The listing builds one solid part. Answer for the finished solid, in the listing's coordinates (mm). A direction names the side the tool comes from. Coordinates: 2 decimals unless noted, no trailing zeros. Loops run counter-clockwise (first coordinate to the right, second up) from the corner with the lowest first, then second, coordinate; pieces in that order, holes last. Notation, with made-up numbers: M 64.25,-20.5 L 94.25,-20.5 A6 ccw 94.25,-13.5 Z; hole C 83,63.5 d10. An arc over 180 degrees is marked long. Return JSON: item names as keys, results as strings. Group by question number.
1. Section B-B (z = -2.25) is taken. Count the separate pieces of the cut face and the enclosed holes in it, then the cut area to 3 significant figures.
2. Section A-A (y = 5.5) is taken. Write down the section's boundary in (x, z), then the cut area to 3 significant figures.
3. Given P1, Ø6, axis at x = -1, y = 7, coming from the -Z side; P2, Ø2.5, axis at y = 0, z = -3, coming from the +X side; P3, Ø0.5, axis at x = 7, z = -2, coming from the +Y side, each flat-ended and moving along its own axis, determine where each tip first touches the part or whether it passes through.
4. Straight lines are drawn through the part: L1, parallel to X at y = 2, z = -0.25; L2, parallel to Y at x = 6.25, z = 0.5; L3, parallel to X at y = 0.5, z = -0.5. For each, find the intervals that lie inside material, in ascending order. Write a range as from..to.
5. Section D-D (z = 1.25) is taken. Write down the section's boundary in (x, y), then the cut area to 3 significant figures.
6. Which of the six approach directions +Z, -Z, +X, -X, +Y, -Y give full straight-line access (tool end or side, diameter ignored) to faces 1 (the face through (-4, 0, -1)), 2 (the face through (0, 0, 2.5))?
7. The mould has two halves that part along X. Classify faces 3 (the face through (1.143, 1.121, -6.207)), 4 (the face through (9, -0.1, 0.4)), 5 (the face through (-1.121, 1.143, -6.207)): pulls with the +X half, pulls with the -X half, needs draft (parallel to the pull), parting line crosses it, or undercut.
```python
from build123d import *

# Parameters (mm, degrees)
SKETCH1_W               = 20
SKETCH1_H               = 20
BOSS_EXTRUDE1_DEPTH     = 2.5
BOSS_EXTRUDE1_TAPER     = 15
SKETCH2_W               = 18
SKETCH2_H               = 18
CUT_EXTRUDE1_DEPTH      = 0.85
SKETCH3_R               = 2
BOSS_EXTRUDE2_DEPTH     = 8.2
BOSS_EXTRUDE2_TAPER     = 1.5
CHAMFER1_SIZE           = 2
CHAMFER1_SIZE_2         = 0.5
FILLET1_R               = 0.5
SKETCH4_W               = 0.5
SKETCH4_H               = 6.160058372
SKETCH4_W_2             = 6.292216955
SKETCH4_H_2             = 0.5
CUT_EXTRUDE_THIN1_DEPTH = 8.2
CUT_EXTRUDE_THIN1_TAPER = 1
BOSS_EXTRUDE3_DEPTH     = 5
FILLET2_R               = 1
FILLET3_R               = 0.75
CUT_EXTRUDE2_DEPTH      = 5
FILLET2_OF_MIRROR1_R    = 1
FILLET3_OF_MIRROR1_R    = 0.75


with BuildPart() as part:
    # Sketch1 → Boss-Extrude1 (new body)
    with BuildSketch(Plane.XY):
        Rectangle(SKETCH1_W, SKETCH1_H)
    extrude(amount=BOSS_EXTRUDE1_DEPTH, taper=BOSS_EXTRUDE1_TAPER)

    # Sketch2 → Cut-Extrude1 (cut)
    with BuildSketch(Plane(origin=(0, 0, 0), x_dir=(-1, 0, 0), z_dir=(0, 0, -1))):
        Rectangle(SKETCH2_W, SKETCH2_H)
    extrude(amount=-CUT_EXTRUDE1_DEPTH, mode=Mode.SUBTRACT)

    # Sketch3 → Boss-Extrude2 (add)
    with BuildSketch(Plane(origin=(0, 0, 0.85), x_dir=(-1, 0, 0), z_dir=(0, 0, -1))):
        Circle(SKETCH3_R)
    extrude(amount=BOSS_EXTRUDE2_DEPTH, taper=BOSS_EXTRUDE2_TAPER)

    # Chamfer1
    # the kernel refuses this chamfer: 2, 0.5 mm, written as the material it takes off along each edge
    with BuildSketch(Plane(origin=(0, 0, -7.35), x_dir=(-1, 0, 0), z_dir=(0, 1, 0))) as chamfer1_piece_1:
        Polygon((1.785275443 + CHAMFER1_SIZE * 0.0261769483079, CHAMFER1_SIZE * 0.999657324976), (1.785275443 - CHAMFER1_SIZE_2, 0), (1.785275443, 0), align=None)
    revolve(axis=Axis((0, 0, -7.35), (0, 0, 1)), mode=Mode.SUBTRACT)

    # Fillet1
    fillet1_edges = [part.edges().sort_by_distance(p)[0] for p in [
        (1.285275443, 0, -7.35),
        (1.83762934, 0, -5.35068535),
    ]]
    fillet(fillet1_edges, radius=FILLET1_R)

    # Sketch4 → Cut-Extrude-Thin1 (cut)
    with BuildSketch(Plane(origin=(0, 0, -7.35), x_dir=(-1, 0, 0), z_dir=(0, 0, -1))):
        with Locations((0, 0.055971591)):
            Rectangle(SKETCH4_W, SKETCH4_H)
        with Locations((0.111262179, 0)):
            Rectangle(SKETCH4_W_2, SKETCH4_H_2)
    extrude(amount=-CUT_EXTRUDE_THIN1_DEPTH, taper=CUT_EXTRUDE_THIN1_TAPER, mode=Mode.SUBTRACT)

    # Sketch5 → Boss-Extrude3 (add)
    with BuildSketch(Plane(origin=(0, 0, 0.85), x_dir=(-1, 0, 0), z_dir=(0, 0, -1))):
        Polygon((4, 2.8), (4, -2.8), (6, -5.15), (8, -5.15), (8, 5.15), (6, 5.15), align=None)
    boss_extrude3 = extrude(amount=BOSS_EXTRUDE3_DEPTH)

    # Fillet2
    fillet2_edges = [part.edges().sort_by_distance(p)[0] for p in [
        (-6, -5.15, -1.65),
        (-6, 5.15, -1.65),
        (-4, 2.8, -1.65),
        (-4, -2.8, -1.65),
    ]]
    fillet(fillet2_edges, radius=FILLET2_R)

    # Fillet3
    fillet3_edges = [part.edges().sort_by_distance(p)[0] for p in [
        (-8, 0, -4.15),
        (-7.231032941, 5.15, -4.15),
        (-4.969493552, 3.939154923, -4.15),
        (-7.231032941, -5.15, -4.15),
        (-4, 0, -4.15),
        (-4.969493552, -3.939154923, -4.15),
        (-4.061506689, -2.777370003, -4.15),
        (-6.042613043, -5.057777128, -4.15),
        (-4.061506689, 2.777370003, -4.15),
        (-6.042613043, 5.057777128, -4.15),
    ]]
    fillet(fillet3_edges, radius=FILLET3_R)

    # Sketch6 → Cut-Extrude2 (cut)
    with BuildSketch(Plane(origin=(0, 0, -4.15), x_dir=(-1, 0, 0), z_dir=(0, 0, -1))):
        Polygon((7, -4.15), (7, 4.15), (6.462065883, 4.15), (5, 2.432072588), (5, -2.432072588), (6.462065883, -4.15), align=None)
    cut_extrude2 = extrude(amount=-CUT_EXTRUDE2_DEPTH, mode=Mode.SUBTRACT)

    # Mirror1: Boss-Extrude3, Cut-Extrude2 across plane
    add(boss_extrude3.mirror(Plane(origin=(0, 0, 0), x_dir=(0, 0, 1), z_dir=(1, 0, 0))))
    add(cut_extrude2.mirror(Plane(origin=(0, 0, 0), x_dir=(0, 0, 1), z_dir=(1, 0, 0))), mode=Mode.SUBTRACT)

    # Fillet2 of Mirror1
    fillet2_of_mirror1_edges = [part.edges().sort_by_distance(p)[0] for p in [
        (6, -5.15, -1.65),
        (6, 5.15, -1.65),
        (4, 2.8, -1.65),
        (4, -2.8, -1.65),
    ]]
    fillet(fillet2_of_mirror1_edges, radius=FILLET2_OF_MIRROR1_R)

    # Fillet3 of Mirror1
    fillet3_of_mirror1_edges = [part.edges().sort_by_distance(p)[0] for p in [
        (8, 0, -4.15),
        (7.231032941, 5.15, -4.15),
        (4.969493552, 3.939154923, -4.15),
        (7.231032941, -5.15, -4.15),
        (4, 0, -4.15),
        (4.969493552, -3.939154923, -4.15),
        (4.061506689, -2.777370003, -4.15),
        (6.042613043, -5.057777128, -4.15),
        (4.061506689, 2.777370003, -4.15),
        (6.042613043, 5.057777128, -4.15),
    ]]
    fillet(fillet3_of_mirror1_edges, radius=FILLET3_OF_MIRROR1_R)


solid = part.part
```
Worked out:
{
 "1": {"separate pieces": "6", "enclosed holes": "2", "area": "53.8 mm^2"},
 "2": {"outline": "M -10,0 L -9,0 L -9,0.85 L 9,0.85 L 9,0 L 10,0 L 9.33,2.5 L -9.33,2.5 Z", "area": "33.0 mm^2"},
 "3": {"P1": "z = 0", "P2": "x = 8", "P3": "y = 5.15"},
 "4": {"L1": "-8..-7, -5..-4, 4..5, 7..8", "L2": "-9.87..-9, -5.13..-3.9, 3.9..5.13, 9..9.87", "L3": "-8..-7, -5..-4, -1.9..-0.13, 0.13..1.9, 4..5, 7..8"},
 "5": {"outline": "M -9.67,-9.67 L 9.67,-9.67 L 9.67,9.67 L -9.67,9.67 Z", "area": "374 mm^2"},
 "6": {"face 1": "-Z", "face 2": "+Z, +X, -X, +Y, -Y"},
 "7": {"face 3": "pulls with the +X half", "face 4": "undercut", "face 5": "pulls with the -X half"}
}
